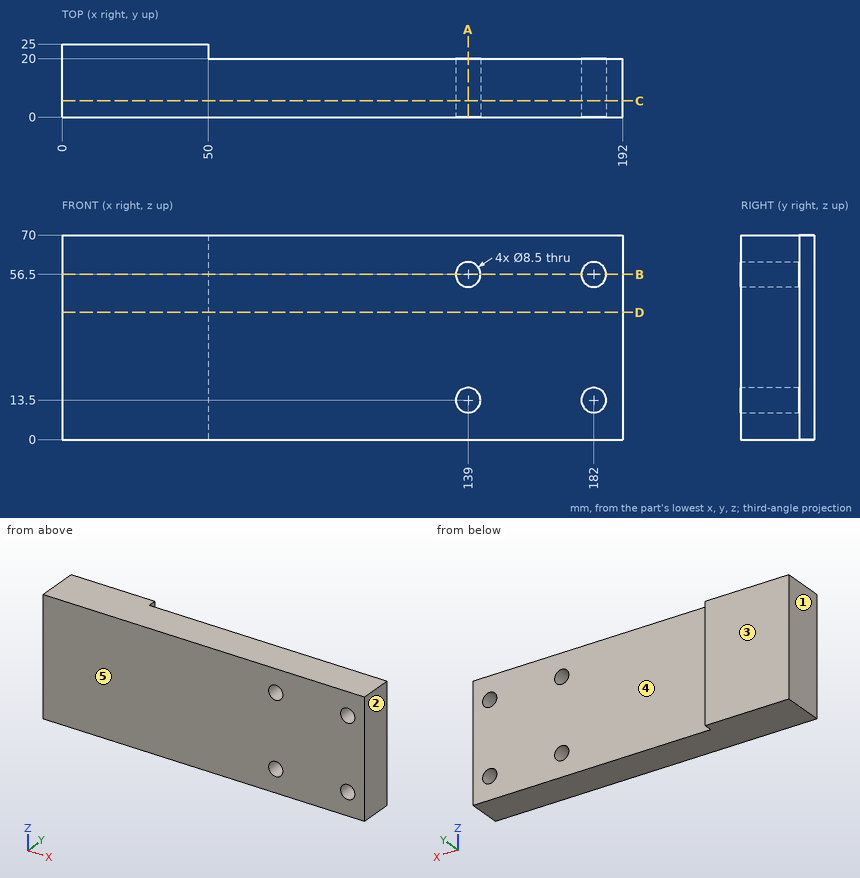
Design review of the part shown in the three views and the two pictorial views. Dimensions are in mm from the part's minimum x, y and z. A direction names the side the tool comes from. Give positions to 0.01 mm unless a question says otherwise; leave off trailing zeros. Loops run counter-clockwise (first coordinate to the right, second up) from the corner with the lowest first, then second, coordinate; pieces in that order, holes last. Notation, with made-up numbers: M 6,60.25 L 10,60.25 A26 ccw 10,90.25 Z; hole C -28,76.25 d4. An arc over 180 degrees is marked long. Write item = value, one per line.
Q1. We need section D-D (z = 43.5). Give the boundary of the cut face in (x, y), plus the area to 3 significant figures.
Output values:
outline = M 0,0 L 192,0 L 192,20 L 50,20 L 50,25 L 0,25 Z
area = 4,090 mm^2
Q2. We need section C-C (y = 5.5). Give the boundary of the cut face in (x, z).
Output values:
outline = M 0,0 L 192,0 L 192,70 L 0,70 Z; hole C 139,13.5 d8.5; hole C 139,56.5 d8.5; hole C 182,13.5 d8.5; hole C 182,56.5 d8.5
Q3. We need section B-B (z = 56.5). Give the boundary of the cut face in (x, y), plus the area to 3 significant figures.
Output values:
outline = M 0,0 L 134.75,0 L 134.75,20 L 50,20 L 50,25 L 0,25 Z; M 143.25,0 L 177.75,0 L 177.75,20 L 143.25,20 Z; M 186.25,0 L 192,0 L 192,20 L 186.25,20 Z
area = 3,750 mm^2
Q4. We need section A-A (x = 139). Give the boundary of the cut face in (y, z), plus the area to 3 significant figures.
Output values:
outline = M 0,0 L 20,0 L 20,9.25 L 0,9.25 Z; M 0,17.75 L 20,17.75 L 20,52.25 L 0,52.25 Z; M 0,60.75 L 20,60.75 L 20,70 L 0,70 Z
area = 1,060 mm^2
Q5. Draft analysis for pull direction X (two halves, no side actions). For the marked faces 1, 2 and 3, state which applies: +X half, -X half, draft (parallel to the pull), parting line (faces both ways), or undercut.
Output values:
face_1 = -X half
face_2 = +X half
face_3 = draft
Q6. For the marked faces 4 and 5, list the 3-axis set-ups (+Z, -Z, +X, -X, +Y, -Y) from which the entire face can be reached by the end or side of a thin tool; tool diameter is ignored.
Output values:
face_4 = +Z, -Z, +X, +Y
face_5 = +Z, -Z, +X, -X, -Y
Q7. Insertion check: pin 1 (5 mm diameter, centred on x = 36.5, z = 12, fed in from -Y); pin 2 (5 mm diameter, centred on x = 182, z = 56.5, fed in from -Y); pin 3 (1.5 mm diameter, centred on x = 52, z = 24.5, fed in from +Y). Each pin has a flat end and moves straight along its axis. Give the tip position at first contact, or say it passes through.
Output values:
pin_1 = 0
pin_2 = through
pin_3 = 20
Q8. To check wall thickness, follow line 1 (X direction, y = 11.5, z = 56.5); line 2 (Z direction, x = 139, y = 7.75); line 3 (X direction, y = 18, z = 55.5). State the ranges of each line that lie inside material, in increasing order. Write a range as [from, to].
Output values:
line_1 = [0, 134.75], [143.25, 177.75], [186.25, 192]
line_2 = [0, 9.25], [17.75, 52.25], [60.75, 70]
line_3 = [0, 134.87], [143.13, 177.87], [186.13, 192]
